Design review of the part built by this model. Coordinates are the model's own, in mm. Give positions to 0.01 mm unless a question says otherwise; leave off trailing zeros. Order: outer loops, then holes, each group sorted by start corner. A loop starts at its lowest first (then second) coordinate and runs counter-clockwise, first axis right, second up. Notation, with made-up numbers: (80, 63) -> (120, 63) arc R25 cw to (120, 95) -> close; hole circle Ø5 at (46, 84). An arc over 180 degrees is marked (long way). Answer in a Markdown table with one row per item. Add a question column.
```python
from build123d import *

# Parameters (mm, degrees)
SKETCH2_W           = 58
SKETCH2_H           = 30
BOSS_EXTRUDE1_DEPTH = 18.7
FILLET1_R           = 10
FILLET2_R           = 1


with BuildPart() as part:
    # Sketch2 → Boss-Extrude1 (new body)
    with BuildSketch(Plane(origin=(0, 0, 0), x_dir=(0, 0, -1), z_dir=(1, 0, 0))):
        Rectangle(SKETCH2_W, SKETCH2_H)
    extrude(amount=BOSS_EXTRUDE1_DEPTH)

    # Fillet1
    # the kernel refuses this fillet: 10 mm, written as the material it takes off along each edge
    with BuildSketch(Plane(origin=(0, -40, 29), x_dir=(1, 0, 0), z_dir=(0, 1, 0))) as fillet1_piece_1:
        with BuildLine():
            CenterArc((FILLET1_R, FILLET1_R), FILLET1_R, 180, 90)
            Line((0, FILLET1_R), (0, 0))
            Line((0, 0), (FILLET1_R, 0))
        make_face()
    extrude(amount=80, mode=Mode.SUBTRACT)
    with BuildSketch(Plane(origin=(18.7, -40, 29), x_dir=(-1, 0, 0), z_dir=(0, 1, 0))) as fillet1_piece_2:
        with BuildLine():
            CenterArc((FILLET1_R, -FILLET1_R), FILLET1_R, 90, 90)
            Line((0, -FILLET1_R), (0, 0))
            Line((0, 0), (FILLET1_R, 0))
        make_face()
    extrude(amount=80, mode=Mode.SUBTRACT)

    # Fillet2
    # the kernel refuses this fillet: 1 mm, written as the material it takes off along each edge
    with BuildSketch(Plane(origin=(1, -14, -28), x_dir=(0, 0, -1), z_dir=(-1, 0, 0))) as fillet2_piece_1_section:
        Polygon((0, 0), (FILLET2_R, 0), (FILLET2_R, FILLET2_R), (0, FILLET2_R), align=None)
    fillet2_piece_1 = extrude(amount=FILLET2_R, mode=Mode.PRIVATE)
    fillet2_piece_1 = fillet2_piece_1 - Plane(origin=(1, -14, -28), x_dir=(0, 0.7071067811865475, 0.7071067811865475), z_dir=(-1, 0, 0)) * Sphere(FILLET2_R, mode=Mode.PRIVATE)
    add(fillet2_piece_1, mode=Mode.SUBTRACT)
    with BuildSketch(Plane(origin=(17.7, -14, -28), x_dir=(1, 0, 0), z_dir=(0, 0, -1))) as fillet2_piece_2_section:
        Polygon((0, 0), (FILLET2_R, 0), (FILLET2_R, FILLET2_R), (0, FILLET2_R), align=None)
    fillet2_piece_2 = extrude(amount=FILLET2_R, mode=Mode.PRIVATE)
    fillet2_piece_2 = fillet2_piece_2 - Plane(origin=(17.7, -14, -28), x_dir=(-0.7071067811865475, 0.7071067811865475, 0), z_dir=(0, 0, -1)) * Sphere(FILLET2_R, mode=Mode.PRIVATE)
    add(fillet2_piece_2, mode=Mode.SUBTRACT)
    with BuildSketch(Plane(origin=(1, 14, -28), x_dir=(-1, 0, 0), z_dir=(0, 1, 0))) as fillet2_piece_3_section:
        Polygon((0, 0), (FILLET2_R, 0), (FILLET2_R, -FILLET2_R), (0, -FILLET2_R), align=None)
    fillet2_piece_3 = extrude(amount=FILLET2_R, mode=Mode.PRIVATE)
    fillet2_piece_3 = fillet2_piece_3 - Plane(origin=(1, 14, -28), x_dir=(0.7071067811865475, 0, 0.7071067811865475), z_dir=(0, 1, 0)) * Sphere(FILLET2_R, mode=Mode.PRIVATE)
    add(fillet2_piece_3, mode=Mode.SUBTRACT)
    with BuildSketch(Plane(origin=(17.7, 14, -28), x_dir=(0, 0, -1), z_dir=(0, 1, 0))) as fillet2_piece_4_section:
        Polygon((0, 0), (FILLET2_R, 0), (FILLET2_R, -FILLET2_R), (0, -FILLET2_R), align=None)
    fillet2_piece_4 = extrude(amount=FILLET2_R, mode=Mode.PRIVATE)
    fillet2_piece_4 = fillet2_piece_4 - Plane(origin=(17.7, 14, -28), x_dir=(-0.7071067811865475, 0, 0.7071067811865475), z_dir=(0, 1, 0)) * Sphere(FILLET2_R, mode=Mode.PRIVATE)
    add(fillet2_piece_4, mode=Mode.SUBTRACT)
    with BuildSketch(Plane(origin=(0, -15, -28), x_dir=(0, 1, 0), z_dir=(0, 0, 1)), Plane(origin=(18.7, 15, 19), x_dir=(-1, 0, 0), z_dir=(0, 0, -1))) as fillet2_piece_5:
        with BuildLine():
            CenterArc((FILLET2_R, -FILLET2_R), FILLET2_R, 90, 90)
            Line((0, -FILLET2_R), (0, 0))
            Line((0, 0), (FILLET2_R, 0))
        make_face()
    extrude(amount=47, mode=Mode.SUBTRACT)
    with BuildSketch(Plane(origin=(18.7, -15, -28), x_dir=(0, 1, 0), z_dir=(0, 0, 1)), Plane(origin=(0, 15, 19), x_dir=(1, 0, 0), z_dir=(0, 0, -1))) as fillet2_piece_6:
        with BuildLine():
            CenterArc((FILLET2_R, FILLET2_R), FILLET2_R, 180, 90)
            Line((0, FILLET2_R), (0, 0))
            Line((0, 0), (FILLET2_R, 0))
        make_face()
    extrude(amount=47, mode=Mode.SUBTRACT)
    with BuildSketch(Plane(origin=(8.7, -15, 19), x_dir=(1, 0, 0), z_dir=(0, 0, -1))) as fillet2_piece_7:
        with BuildLine():
            CenterArc((10 - FILLET2_R, -FILLET2_R), FILLET2_R, 0, 90)
            Line((10 - FILLET2_R, 0), (10, 0))
            Line((10, 0), (10, -FILLET2_R))
        make_face()
    revolve(axis=Axis((8.7, -15, 19), (0, -1, 0)), revolution_arc=100.602378983, mode=Mode.SUBTRACT)
    with BuildSketch(Plane(origin=(10, -15, 19), x_dir=(0.1839921630034736, 0, 0.9829277104412629), z_dir=(0.9829277104412629, 0, -0.1839921630034736))) as fillet2_piece_8:
        with BuildLine():
            CenterArc((10 - FILLET2_R, -FILLET2_R), FILLET2_R, 0, 90)
            Line((10 - FILLET2_R, 0), (10, 0))
            Line((10, 0), (10, -FILLET2_R))
        make_face()
    revolve(axis=Axis((10, -15, 19), (0, -1, 0)), revolution_arc=100.602378983, mode=Mode.SUBTRACT)
    with BuildSketch(Plane(origin=(8.7, 15, 19), x_dir=(1, 0, 0), z_dir=(0, 0, -1))) as fillet2_piece_9:
        with BuildLine():
            CenterArc((10 - FILLET2_R, FILLET2_R), FILLET2_R, 270, 90)
            Line((10, FILLET2_R), (10, 0))
            Line((10, 0), (10 - FILLET2_R, 0))
        make_face()
    revolve(axis=Axis((8.7, 15, 19), (0, -1, 0)), revolution_arc=100.602378983, mode=Mode.SUBTRACT)
    with BuildSketch(Plane(origin=(10, 15, 19), x_dir=(0.1839921630034736, 0, 0.9829277104412629), z_dir=(0.9829277104412629, 0, -0.1839921630034736))) as fillet2_piece_10:
        with BuildLine():
            CenterArc((10 - FILLET2_R, FILLET2_R), FILLET2_R, 270, 90)
            Line((10, FILLET2_R), (10, 0))
            Line((10, 0), (10 - FILLET2_R, 0))
        make_face()
    revolve(axis=Axis((10, 15, 19), (0, -1, 0)), revolution_arc=100.602378983, mode=Mode.SUBTRACT)
    with BuildSketch(Plane(origin=(0, 14, -29), x_dir=(0, 0, 1), z_dir=(0, -1, 0)), Plane(origin=(18.7, 14, -29), x_dir=(-1, 0, 0), z_dir=(0, -1, 0))) as fillet2_piece_11:
        with BuildLine():
            CenterArc((FILLET2_R, -FILLET2_R), FILLET2_R, 90, 90)
            Line((0, -FILLET2_R), (0, 0))
            Line((0, 0), (FILLET2_R, 0))
        make_face()
    extrude(amount=28, mode=Mode.SUBTRACT)
    with BuildSketch(Plane(origin=(1, -15, -29), x_dir=(0, 1, 0), z_dir=(1, 0, 0)), Plane(origin=(1, 15, -29), x_dir=(0, 0, 1), z_dir=(1, 0, 0))) as fillet2_piece_12:
        with BuildLine():
            CenterArc((FILLET2_R, FILLET2_R), FILLET2_R, 180, 90)
            Line((0, FILLET2_R), (0, 0))
            Line((0, 0), (FILLET2_R, 0))
        make_face()
    extrude(amount=16.7, mode=Mode.SUBTRACT)


solid = part.part
```
1) Clearance check with a flat-ended pin moving along its axis: P1, Ø1, axis at y = 10, z = 22.5, coming from the -X side. State where the tip first meets the part, or that it passes through.
2) For L1, parallel to Z at x = 9.25, y = 0; L2, parallel to X at y = 10, z = 25.5; L3, parallel to Z at x = 11.25, y = -2, list the stretches that pass through material, from the lowest coordinate up.
3) Add section A-A, the plane y = 6.5. Write out the cut boundary in (x, z), and give its area (3 significant figures).
Verdict:
| question | item | result |
|---|---|---|
| 1 | P1 | stops at x = 0.46 |
| 2 | L1 | z = -29 to 28.97 |
| 2 | L2 | x = 2.4 to 16.3 |
| 2 | L3 | z = -29 to 28.67 |
| 3 | outline | (0, -28) arc R1 ccw to (1, -29) -> (17.7, -29) arc R1 ccw to (18.7, -28) -> (18.7, 19) arc R10 ccw to (9.35, 28.98) arc R10 ccw to (0, 19) -> close |
| 3 | area | 1,040 mm2 |
